Could you check a few things on this model? Use its own coordinates, in mm. A direction names the side the tool comes from. Give positions to 0.01 mm unless a question says otherwise; leave off trailing zeros. Write each loop counter-clockwise with the first axis right and the second up, starting at its lowest first coordinate (ties: lowest second). Pieces come first, ordered by that corner, then holes. Notation, with made-up numbers: M 62.5,24.25 L 73.5,24.25 A15 cw 73.5,50.25 Z; hole C 59.5,55 d10. An arc over 180 degrees is marked long. Use one line per item in the form item = value.
from build123d import *

# Parameters (mm, degrees)
F2_R     = 1.55
F3_DEPTH = 15
F5_DEPTH = 13


with BuildPart() as f1:
    # F0 (on Front) → F1 (revolve)
    with BuildSketch(Plane.XZ):
        Polygon((-29.132355, 2.5), (-29.132355, 0), (0, 0), (0, 1.699776), (-14.132355, 2.5), align=None)
    revolve(axis=Axis((-14.566178, 0, 0), (-1, 0, 0)))

    # F2 (on Right) → F3 (cut)
    with BuildSketch(Plane.YZ):
        Circle(F2_R)
    extrude(amount=-F3_DEPTH, mode=Mode.SUBTRACT)

    # F4 (on face) → F5 (cut)
    with BuildSketch(Plane(origin=(-29.132355, 0, 0), x_dir=(0, -1, 0), z_dir=(-1, 0, 0))):
        Polygon((-2.934946, 0.25), (-2.934946, 0), (-2.934946, -0.25), (-0.25, -0.25), (-0.25, -2.634228), (0.25, -2.634228), (0.25, -0.25), (3.675647, -0.25), (3.675647, 0.25), (0.25, 0.25), (0.25, 2.968905), (-0.25, 2.968905), (-0.25, 0.25), align=None)
    extrude(amount=-F5_DEPTH, mode=Mode.SUBTRACT)


solid = f1.part
1) If I drill on L1, parallel to Y at x = -8.25, z = -0.05; L2, parallel to Z at x = -16.25, y = -1.9; L3, parallel to Z at x = -2, y = -1.15, over which ranges is the centre line in solid material (lowest first)?
Checked values:
L1 = -2.17 to -1.55, 1.55 to 2.17
L2 = -1.62 to -0.25, 0.25 to 1.62
L3 = -1.4 to -1.04, 1.04 to 1.4
2) I want a section at A-A, the plane x = -25.75. Please give me the cut outline in (y, z), plus the area to 3 significant figures.
Checked values:
outline = M -2.49,-0.25 A2.5 ccw -0.25,-2.49 L -0.25,-0.25 Z; M -2.49,0.25 L -0.25,0.25 L -0.25,2.49 A2.5 ccw Z; M 0.25,-2.49 A2.5 ccw 2.49,-0.25 L 0.25,-0.25 Z; M 0.25,0.25 L 2.49,0.25 A2.5 ccw 0.25,2.49 Z
area = 14.9 mm2
3) For pin 1 Ø3 at (x, y) = (-25.5, -1.5) entering from +Z; pin 2 Ø1.8 at (x, z) = (-23, -1) entering from +Y; pin 3 Ø1.1 at (x, y) = (-23, 2) entering from -Z, each with a flat end and sliding along its axis, tell me the tip position at first contact or that it passes through.
Checked values:
pin_1 = 2.49
pin_2 = 2.49
pin_3 = -2.04
4) I want a section at B-B, the plane y = 0. Please give me the cut outline in (x, z), plus the area to 3 significant figures.
Checked values:
outline = M -16.13,-2.5 L -14.13,-2.5 L 0,-1.7 L 0,-1.55 L -15,-1.55 L -15,1.55 L 0,1.55 L 0,1.7 L -14.13,2.5 L -16.13,2.5 Z
area = 22.9 mm2
5) For faces 4 (the flat face through (-29.132, -1, 1)), 5 (the flat face through (-23, -0.25, 1)), 6 (the flat face through (-23, -1, -0.25)), 7 (the cylindrical face through (-7.395, 0.715, -1.375)), which set-ups out of +Z, -Z, +X, -X, +Y, -Y let a thin tool reach every point of the face, with its end or its side?
Checked values:
face_4 = +Z, -Z, -X, +Y, -Y
face_5 = +Z, -Z, -X
face_6 = -X, +Y, -Y
face_7 = +X
6) Thinking about a two-plate mould opening in Y: for faces 1 (the flat face through (-23, -0.25, -1)), 2 (the flat face through (-29.132, 1, -1)), 3 (the cylindrical face through (-21.737, 0.751, 2.385)), which applies, released by +Y, released by -Y, zero draft, split by the parting line, or undercut?
Checked values:
face_1 = undercut
face_2 = zero draft
face_3 = split by the parting line
7) I want a section at D-D, the plane x = -11. Please give me the cut outline in (y, z), plus the area to 3 significant figures.
Checked values:
outline = C 0,0 d4.65; hole C 0,0 d3.1
area = 9.40 mm2
